from build123d import *

# Parameters (mm, degrees)
SKETCH2_R           = 7.9375
SKETCH2_R_2         = 3.2639
SKETCH2_R_3         = 4.191
BOSS_EXTRUDE1_DEPTH = 3.175
FILLET1_R           = 2.54
FILLET2_R           = 3.81
FILLET3_R           = 1.905
FILLET4_R           = 6.35


with BuildPart() as part:
    # Sketch2 → Boss-Extrude1 (new body)
    with BuildSketch(Plane.XY):
        with BuildLine():
            ThreePointArc((54.035830718, 67.22198524), (46.333024889, 72.662028043), (40.750647472, 65.061742146))
            ThreePointArc((40.750647472, 65.061742146), (31.550758366, 30.452598432), (0.230104832, 13.090356345))
            Line((0.230104832, 13.090356345), (0.171615761, 13.016368706))
            ThreePointArc((0.171615761, 13.016368706), (-13.004550196, -0.580500165), (1.330677778, -12.949308974))
            Line((1.330677778, -12.949308974), (46.572932, -8.300191215))
            ThreePointArc((46.572932, -8.300191215), (51.37742802, -6.133039654), (53.924522362, -1.518709983))
            ThreePointArc((53.924522362, -1.518709983), (57.106411985, 32.846575472), (54.035830718, 67.22198524))
        make_face()
        Circle(SKETCH2_R, mode=Mode.SUBTRACT)
        with BuildLine():
            ThreePointArc((9.848859751, 8.512066016), (23.445327069, 14.632175726), (34.749899024, 24.354640398))
            Line((34.749899024, 24.354640398), (40.595697266, 6.584997244))
            ThreePointArc((40.595697266, 6.584997244), (37.546758205, 1.678923993), (38.414831114, -4.031770672))
            Line((38.414831114, -4.031770672), (11.074870198, -6.841239387))
            ThreePointArc((11.074870198, -6.841239387), (12.976194182, 1.036190528), (9.848859751, 8.512066016))
        make_face(mode=Mode.SUBTRACT)
        with Locations((45.72, 0)):
            Circle(SKETCH2_R_2, mode=Mode.SUBTRACT)
        with BuildLine():
            Line((45.933946154, 8.34115665), (38.882442516, 29.775817606))
            ThreePointArc((38.882442516, 29.775817606), (45.039190515, 42.544935267), (47.523781163, 56.501393309))
            ThreePointArc((47.523781163, 56.501393309), (48.257752726, 32.370804269), (45.933946154, 8.34115665))
        make_face(mode=Mode.SUBTRACT)
        with Locations((47.413333333, 66.018287029)):
            Circle(SKETCH2_R_3, mode=Mode.SUBTRACT)
    extrude(amount=BOSS_EXTRUDE1_DEPTH)

    # Fillet1
    fillet1_edges = [part.edges().sort_by_distance(p)[0] for p in [
        (38.414831114, -4.031770672, 1.5875),
        (9.848859751, 8.512066016, 1.5875),
        (11.074870198, -6.841239387, 1.5875),
    ]]
    fillet(fillet1_edges, radius=FILLET1_R)

    # Fillet2
    fillet2_edges = [part.edges().sort_by_distance(p)[0] for p in [
        (40.595697266, 6.584997244, 1.5875),
        (34.749899024, 24.354640398, 1.5875),
    ]]
    fillet(fillet2_edges, radius=FILLET2_R)

    # Fillet3
    fillet3_edges = [part.edges().sort_by_distance(p)[0] for p in [
        (47.523781163, 56.501393309, 1.5875),
        (45.933946154, 8.34115665, 1.5875),
    ]]
    fillet(fillet3_edges, radius=FILLET3_R)

    # Fillet4
    fillet4_edges = [part.edges().sort_by_distance(p)[0] for p in [
        (38.882442516, 29.775817606, 1.5875),
    ]]
    fillet(fillet4_edges, radius=FILLET4_R)


solid = part.part
Model file for the job. Use its own axes, mm. A direction names the side the tool comes from. Coordinates: 2 decimals unless noted, no trailing zeros. Order: outer loops, then holes, each group sorted by start corner. A loop starts at its lowest first (then second) coordinate and runs counter-clockwise, first axis right, second up. Notation, with made-up numbers: (5.5, -21.5) -> (9.5, -21.5) arc R25 cw to (9.5, 12.5) -> close; hole circle Ø7 at (61.25, 73). An arc over 180 degrees is marked (long way). Return JSON: item names as keys, results as strings. Group by question number.
Item 1: Saw through at D-D on y = 44.5. Write the cut outline in (x, z) (3 decimals), then the cut area to 3 significant figures.
Item 2: Flat gauge pins, fed straight in: P1, Ø1.5, axis at y = -1, z = 2.5, coming from the -X side; P2, Ø1.5, axis at y = 42.5, z = 1.5, coming from the +X side; P3, Ø1.5, axis at x = 19, z = 1, coming from the +Y side. Where does each tip first touch, or does it go through?
Item 3: Pull direction Y, two halves, no side cores. Call faces 3 (the cylindrical face through (51.322, -6.184, 1.565)), 4 (the flat face through (30, 21, 3.175)), 5 (the flat face through (38.263, 13.674, 1.565)): pulls with the +Y half, pulls with the -Y half, needs draft (parallel to the pull), parting line crosses it, or undercut.
Item 4: Tool access for faces 1 (the cylindrical face through (31.865, 30.861, 1.565)), 2 (the cylindrical face through (45.405, 14.843, 1.61)): list every direction of +Z, -Z, +X, -X, +Y, -Y with a clear straight run to the whole face (end or side of a thin tool).
Item 5: Saw through at B-B on x = -4.5. Write the cut outline in (y, z) (3 decimals), then the cut area to 3 significant figures.
Item 6: Saw through at C-C on z = 2.2. State how many separate pieces and enclosed holes the cut face has, then the cut area to 3 significant figures.
Item 7: Saw through at A-A on y = 24.5. Write the cut outline in (x, z) (3 decimals).
Item 8: Wall check: line 1 along X through (y, z) = (3.5, 1.25); line 2 along Y through (x, z) = (0, 2.5); line 3 along X through (y, z) = (16, 1). Give the ranges that are in metal, low to high. Write a range as [from, to].
Values found:
{
 "1": {"outline": "(38.998, 0) -> (56.769, 0) -> (56.769, 3.175) -> (38.998, 3.175) -> close", "area": "56.4 mm2"},
 "2": {"P1": "stops at x = -13.02", "P2": "stops at x = 56.91", "P3": "stops at y = 19.81"},
 "3": {"face 3": "pulls with the -Y half", "face 4": "needs draft", "face 5": "undercut"},
 "4": {"face 1": "+Z, -Z, -X", "face 2": "+Z, -Z"},
 "5": {"outline": "(-12.215, 0) -> (-6.539, 0) -> (-6.539, 3.175) -> (-12.215, 3.175) -> close; (6.539, 0) -> (12.215, 0) -> (12.215, 3.175) -> (6.539, 3.175) -> close", "area": "36.0 mm2"},
 "6": {"separate pieces": "1", "enclosed holes": "5", "area": "1,850 mm2"},
 "7": {"outline": "(25.989, 0) -> (40.618, 0) -> (40.618, 3.175) -> (25.989, 3.175) -> close; (47.835, 0) -> (56.91, 0) -> (56.91, 3.175) -> (47.835, 3.175) -> close"},
 "8": {"line 1": "x = [-12.54, -7.12], [7.12, 12.54], [38.15, 54.78]", "line 2": "y = [-13.02, -7.94], [7.94, 13.02]", "line 3": "x = [12.19, 25.49], [37.5, 43.42], [46.94, 56.33]"}
}
